Could you check a few things on this model? Use its own coordinates, in mm. A direction names the side the tool comes from. Round coordinates to 2 decimals unless told otherwise and drop trailing zeros. Write each loop counter-clockwise with the first axis right and the second up, starting at its lowest first coordinate (ties: lowest second). Pieces come first, ordered by that corner, then holes. Notation, with made-up numbers: (42.25, 67.5) -> (86.25, 67.5) arc R17 cw to (86.25, 78.5) -> close; hole circle Ø7 at (41, -38.5). An arc over 180 degrees is marked (long way). Return JSON: item names as keys, results as strings.
from build123d import *

# Parameters (mm, degrees)
F2_R      = 6.985
F3_DEPTH  = 8.89
F4_R      = 1.9622727835
F5_R      = 6.985
F6_DEPTH  = 8.89
F7_R      = 1.8396307345
F9_DEPTH  = 5.969
F12_DEPTH = 19.05
F14_DEPTH = 3.175
F15_W     = 57.15
F15_H     = 37.084
F16_DEPTH = 3.175


with BuildPart() as f1:
    # F0 (on Right) → F1 (revolve)
    with BuildSketch(Plane.YZ):
        with BuildLine():
            Line((-12.7, 0), (0, 0))
            Line((0, 0), (0, 50.8))
            ThreePointArc((0, 50.8), (-8.9802561211, 47.0802561211), (-12.7, 38.1))
            Line((-12.7, 38.1), (-12.7, 0))
        make_face()
        with BuildLine():
            Line((0, 50.8), (0, 0))
            Line((0, 0), (12.7, 0))
            Line((12.7, 0), (12.7, 38.1))
            ThreePointArc((12.7, 38.1), (8.9802561211, 47.0802561211), (0, 50.8))
        make_face()
    revolve(axis=Axis((0, -14.7607661784, 0), (0, -1, 0)))

    # F2 (on face) → F3 (join)
    with BuildSketch(Plane.XZ.offset(12.7)):
        Circle(F2_R)
    extrude(amount=F3_DEPTH)

    # F4
    f4_edges = [f1.edges().sort_by_distance(p)[0] for p in [
        (-6.985, -21.59, 0),
    ]]
    fillet(f4_edges, radius=F4_R)

    # F5 (on face) → F6 (join)
    with BuildSketch(Plane(origin=(0, 12.7, 0), x_dir=(-1, 0, 0), z_dir=(0, 1, 0))):
        Circle(F5_R)
    extrude(amount=F6_DEPTH)

    # F7
    f7_edges = [f1.edges().sort_by_distance(p)[0] for p in [
        (6.985, 21.59, 0),
    ]]
    fillet(f7_edges, radius=F7_R)

    # F8 (on face) → F9 (join)
    with BuildSketch(Plane.XZ.offset(12.7)):
        with BuildLine():
            Line((1.7471951485, 62.4704148293), (0, 62.4704148293))
            Line((0, 62.4704148293), (-12.7, 62.4704148293))
            Line((-12.7, 62.4704148293), (-38.1, 62.4704148293))
            Line((-38.1, 62.4704148293), (-38.1, 53.124037792))
            ThreePointArc((-38.1, 53.124037792), (-37.1499121134, 50.6066973892), (-34.7734893943, 49.3448397282))
            Line((-34.7734893943, 49.3448397282), (-18.2441843429, 47.2301731899))
            ThreePointArc((-18.2441843429, 47.2301731899), (-14.2834798111, 45.1270770883), (-12.7, 40.9315097502))
            Line((-12.7, 40.9315097502), (-12.7, 0))
            Line((-12.7, 0), (-12.7, -3.81))
            ThreePointArc((-12.7, -3.81), (-10.8401280605, -8.3001280605), (-6.35, -10.16))
            Line((-6.35, -10.16), (9.0258122236, -10.16))
            ThreePointArc((9.0258122236, -10.16), (10.9539405401, -9.8601918313), (12.7, -8.9890775418))
            Line((12.7, -8.9890775418), (12.7, 0))
            Line((12.7, 0), (12.7, 62.4704148293))
            Line((12.7, 62.4704148293), (1.7471951485, 62.4704148293))
        make_face()
        with BuildLine():
            Line((63.5, 62.4704148293), (12.7, 62.4704148293))
            Line((12.7, 62.4704148293), (12.7, 0))
            Line((12.7, 0), (12.7, -8.9890775418))
            ThreePointArc((12.7, -8.9890775418), (13.7247586768, -8.0811125283), (14.531070583, -6.9745900834))
            Line((14.531070583, -6.9745900834), (48.968929417, 52.9350049127))
            ThreePointArc((48.968929417, 52.9350049127), (51.2939870776, 55.2666702377), (54.4741877764, 56.1204148293))
            Line((54.4741877764, 56.1204148293), (63.5, 56.1204148293))
            Line((63.5, 56.1204148293), (63.5, 62.4704148293))
        make_face()
    extrude(amount=F9_DEPTH)


with BuildPart() as f10_1:
    # F10: instance of F1
    add(f1.part.mirror(Plane.XZ))


with BuildPart() as f12:
    # F11 (on face) → F12 (new body)
    with BuildSketch(Plane.XY.offset(62.4704148293)):
        with BuildLine():
            ThreePointArc((63.5, -16.267034341), (67.0473997645, -8.4749308625), (68.2625, 0))
            ThreePointArc((68.2625, 0), (31.597067385, 29.453153883), (10.7415203959, -12.7))
            Line((10.7415203959, -12.7), (63.5, -12.7))
            Line((63.5, -12.7), (63.5, -16.267034341))
        make_face()
        with BuildLine():
            Line((63.5, -12.7), (10.7415203959, -12.7))
            ThreePointArc((10.7415203959, -12.7), (12.4015653576, -15.7913540642), (14.4093933119, -18.669))
            Line((14.4093933119, -18.669), (61.7906066881, -18.669))
            ThreePointArc((61.7906066881, -18.669), (62.6746673631, -17.4889144958), (63.5, -16.267034341))
            Line((63.5, -16.267034341), (63.5, -12.7))
        make_face()
        with BuildLine():
            Line((61.7906066881, -18.669), (14.4093933119, -18.669))
            ThreePointArc((14.4093933119, -18.669), (38.1, -30.1625), (61.7906066881, -18.669))
        make_face()
    extrude(amount=F12_DEPTH)

    # F13 (on face) → F14 (join)
    with BuildSketch(Plane.XY.offset(81.5204148293)):
        with BuildLine():
            Line((-1.5875, -31.75), (77.7875, -31.75))
            ThreePointArc((77.7875, -31.75), (82.2776280605, -29.8901280605), (84.1375, -25.4))
            Line((84.1375, -25.4), (84.1375, 25.4))
            ThreePointArc((84.1375, 25.4), (82.2776280605, 29.8901280605), (77.7875, 31.75))
            Line((77.7875, 31.75), (-1.5875, 31.75))
            ThreePointArc((-1.5875, 31.75), (-6.0776280605, 29.8901280605), (-7.9375, 25.4))
            Line((-7.9375, 25.4), (-7.9375, -25.4))
            ThreePointArc((-7.9375, -25.4), (-6.0776280605, -29.8901280605), (-1.5875, -31.75))
        make_face()
    extrude(amount=-F14_DEPTH)


with BuildPart() as f1_1:
    add(f1.part)

    add(f10_1.part)  # F16 merges F10_1

    add(f12.part)  # F16 merges F12
    # F15 (on face) → F16 (join)
    with BuildSketch(Plane.XY.offset(62.4704148293)):
        with Locations((-9.525, -0.127)):
            Rectangle(F15_W, F15_H)
    extrude(amount=F16_DEPTH)


solid = f1_1.part
1) I want a section at A-A, the plane y = 2. Please give me the cut outline in (x, z).
Return value:
{"outline": "circle Ø101.28 at (0, 0); (-38.1, 62.47) -> (68.2, 62.47) -> (68.2, 78.35) -> (84.14, 78.35) -> (84.14, 81.52) -> (-7.94, 81.52) -> (-7.94, 78.35) -> (8, 78.35) -> (8, 65.65) -> (-38.1, 65.65) -> close"}
2) If I drill on probe 1 along Y at (x, z) = (-25.5, 52); probe 2 along Y at (x, z) = (-5, 42.5); probe 3 along Z at (x, y) = (-5.5, -9), over which ranges is the centre line in solid material (lowest first)? Write a range as [from, to].
Return value:
{"probe 1": "[-18.67, -12.7], [12.7, 18.67]", "probe 2": "[-18.67, -12.7], [-11.8, 11.8], [12.7, 18.67]", "probe 3": "[-46.74, 46.74], [62.47, 65.65], [78.35, 81.52]"}
3) For faces 1 (the face through (-12, 18.415, 64)), 2 (the face through (38, -23, 62.47)), 3 (the face through (59, -16, 56.12)), which set-ups out of +Z, -Z, +X, -X, +Y, -Y let a thin tool reach every point of the face, with its end or its side?
Return value:
{"face 1": "-X, +Y", "face 2": "-Z, +X, -X, -Y", "face 3": "-Z, +X, +Y, -Y"}
4) Thinking about a two-plate mould opening in Z: for faces 4 (the face through (82.23, -29.94, 79.96)), 5 (the face through (0.909, 19.202, 6.926)), 6 (the face through (-14.33, 15.64, 45.18)), which applies, pulls with the +Z half, pulls with the -Z half, needs draft (parallel to the pull), parting line crosses it, or undercut?
Return value:
{"face 4": "needs draft", "face 5": "undercut", "face 6": "pulls with the -Z half"}
5) Will these pins go through, and if not, where does the flat tip stop? pin 1 Ø1 at (x, y) = (25, -16) entering from -Z; pin 2 Ø3 at (x, z) = (24, 22) entering from +Y; pin 3 Ø12 at (x, z) = (37, 46.5) entering from -Y.
Return value:
{"pin 1": "z = 10.37", "pin 2": "y = 18.67", "pin 3": "y = -18.67"}
